Could you check a few things on this model? Use its own coordinates, in mm. Face numbers are marked on the shaded views. A direction names the side the tool comes from. Coordinates: 2 decimals unless noted, no trailing zeros. Write each loop counter-clockwise with the first axis right and the second up, starting at its lowest first coordinate (ties: lowest second). Pieces come first, ordered by that corner, then holes.
```python
from build123d import *

# Parameters (mm, degrees)
SKETCH_W     = 114
SKETCH_H     = 30
SKETCH_R     = 3.25
SKETCH_R_2   = 1.6
SKETCH_R_3   = 3.5
PAD_DEPTH    = 3
SKETCH001_W  = 44.703079
SKETCH001_H  = 47.60326
POCKET_DEPTH = 1


with BuildPart() as part:
    # Sketch → Pad (new body)
    with BuildSketch(Plane.XY):
        Rectangle(SKETCH_W, SKETCH_H)
        with Locations((41, 0)):
            Circle(SKETCH_R, mode=Mode.SUBTRACT)
        with Locations((51, 10)):
            Circle(SKETCH_R_2, mode=Mode.SUBTRACT)
        with Locations((31, 10)):
            Circle(SKETCH_R_2, mode=Mode.SUBTRACT)
        with Locations((31, -10)):
            Circle(SKETCH_R_2, mode=Mode.SUBTRACT)
        with Locations((51, -10)):
            Circle(SKETCH_R_2, mode=Mode.SUBTRACT)
        with Locations((-45, 0)):
            Circle(SKETCH_R_3, mode=Mode.SUBTRACT)
        with Locations((-54.5, 9.5)):
            Circle(SKETCH_R_2, mode=Mode.SUBTRACT)
        with Locations((-21.5, 9.5)):
            Circle(SKETCH_R_2, mode=Mode.SUBTRACT)
        with Locations((-21.5, -9.5)):
            Circle(SKETCH_R_2, mode=Mode.SUBTRACT)
        with Locations((-54.5, -9.5)):
            Circle(SKETCH_R_2, mode=Mode.SUBTRACT)
    extrude(amount=PAD_DEPTH)

    # Sketch001 (on Face16 of Pad) → Pocket (cut)
    with BuildSketch(Plane.XY.offset(3)):
        with Locations((42.35154, 0.341099)):
            Rectangle(SKETCH001_W, SKETCH001_H)
    extrude(amount=-POCKET_DEPTH, mode=Mode.SUBTRACT)


solid = part.part
```
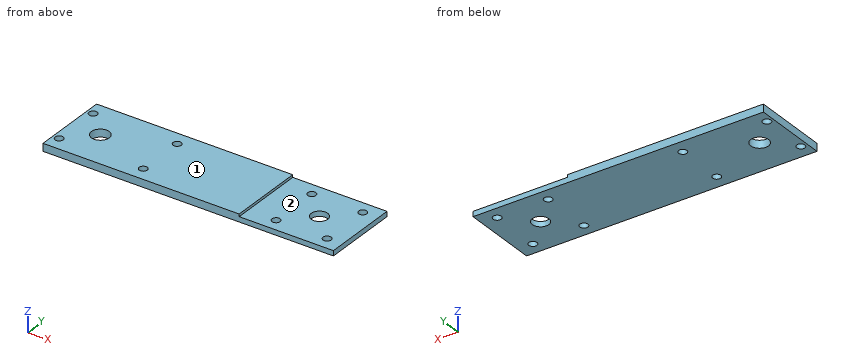
Item 1: Will these pins go through, and if not, where does the flat tip stop? pin 1 Ø4 at (x, y) = (51, 10) entering from +Z; pin 2 Ø2.5 at (x, y) = (-54.5, 9.5) entering from +Z; pin 3 Ø0.5 at (y, z) = (-3.5, 2.5) entering from +X.
Item 2: I want a section at B-B, the plane x = -21.5. List the corners of the cut face in (y, z) for me.
Item 3: I want a section at A-A, the plane x = 41. List the corners of the cut face in (y, z) for me, then the cut area to 3 significant figures.
Item 4: If I drill on line 1 along Y through (x, z) = (-21.5, 0.9); line 2 along Y through (x, z) = (31, 1.1); line 3 along X through (y, z) = (0.25, 1.9), over which ranges is the centre line in solid material (lowest first)?
Item 5: I want a section at D-D, the plane y = 4.5. List the corners of the cut face in (x, z) for me.
Item 6: I want a section at C-C, the plane y = 0. List the corners of the cut face in (x, z) for me, then the cut area to 3 significant figures.
Item 7: Which directions (+Z, -Z, +X, -X, +Y, -Y) give clear straight access to the entire face, cutting with the end or side of a thin tool? Please do the marked faces 1 and 2.
Taken from the geometry:
1. pin 1: stops at z = 2
1. pin 2: passes through
1. pin 3: stops at x = 20
2. outline: (-15, 0) - (-11.1, 0) - (-11.1, 3) - (-15, 3) - close; (-7.9, 0) - (7.9, 0) - (7.9, 3) - (-7.9, 3) - close; (11.1, 0) - (15, 0) - (15, 3) - (11.1, 3) - close
3. outline: (-15, 0) - (-3.25, 0) - (-3.25, 2) - (-15, 2) - close; (3.25, 0) - (15, 0) - (15, 2) - (3.25, 2) - close
3. area: 47.0 mm2
4. line 1: y = -15 to -11.1, -7.9 to 7.9, 11.1 to 15
4. line 2: y = -15 to -11.6, -8.4 to 8.4, 11.6 to 15
4. line 3: x = -57 to -48.49, -41.51 to 37.76, 44.24 to 57
5. outline: (-57, 0) - (57, 0) - (57, 2) - (20, 2) - (20, 3) - (-57, 3) - close
6. outline: (-57, 0) - (-48.5, 0) - (-48.5, 3) - (-57, 3) - close; (-41.5, 0) - (37.75, 0) - (37.75, 2) - (20, 2) - (20, 3) - (-41.5, 3) - close; (44.25, 0) - (57, 0) - (57, 2) - (44.25, 2) - close
6. area: 271 mm2
7. face 1: +Z, +X, -X, +Y, -Y
7. face 2: +Z, +X, +Y, -Y
